Autodesk Inventor part; units mm, degrees
ref_plane "YZ Plane" through (0, 0, 0) normal (1, 0, 0) x (0, 1, 0)
ref_plane "XZ Plane" through (0, 0, 0) normal (0, 1, 0) x (-1, 0, 0)
ref_plane "XY Plane" through (0, 0, 0) normal (0, 0, 1) x (1, 0, 0)
sketch "Szkic1" plane through (0, 0, 0) normal (0, 1, 0) x (-1, 0, 0)
  circle A0 centre (0, 0) radius 10
  dimension "d0" = 20
extrude "Wyciągnięcie proste1" add sketch "Szkic1" along normal mid plane 30
sketch "Szkic2" plane through (0, 15, 0) normal (0, 1, 0) x (1, 0, 0)
  circle A0 centre (0, 0) radius 10
  circle A1 centre (0, 0) radius 15
  dimension "d3" = 30
extrude "Wyciągnięcie proste2" add sketch "Szkic2" along normal blind 5 contours A0 | A1
mirror "Odbicie lustrzane1" about plane through (0, 0, 0) normal (0, 1, 0) of "Wyciągnięcie proste2"
properties part number "RevolvingConnector2" material "Aluminium 6061"
Verification items for the finished model (mm, model axes). A direction names the side the tool comes from. Coordinates: 2 decimals unless noted, no trailing zeros. Write each loop counter-clockwise with the first axis right and the second up, starting at its lowest first coordinate (ties: lowest second). Pieces come first, ordered by that corner, then holes. Notation, with made-up numbers: (39.5, 55) - (55.5, 55) arc R18 cw to (55.5, 85) - close; hole circle Ø6 at (0.5, 68.5). An arc over 180 degrees is marked (long way). Answer as a JSON object with one key per item and string values.
(1) Tool access check on faces 1 (the flat face through (3, 15, 10)), 2 (the cylindrical face through (-14.985, -17.465, -0.66)). Record the directions out of +Z, -Z, +X, -X, +Y, -Y that give a thin tool (end or side, any length) a straight path to the whole face; none if there is none.
Report:
{"face 1": "none", "face 2": "+Y, -Y"}
(2) Cross-section at C-C on z = 0. Record the cut outline in (x, y).
Report:
{"outline": "(-15, -20) - (15, -20) - (15, -15) - (10, -15) - (10, 15) - (15, 15) - (15, 20) - (-15, 20) - (-15, 15) - (-10, 15) - (-10, -15) - (-15, -15) - close"}
(3) Cross-section at D-D on y = -12.5. Record the cut outline in (x, z).
Report:
{"outline": "circle Ø20 at (0, 0)"}
(4) Mould release check, pull along Y, two halves, no side actions. Record for faces 3 (the flat face through (0, 20, 0)), 4 (the flat face through (-3, -15, 10)), 5 (the cylindrical face through (-14.985, 17.465, 0.66)): pulls with the +Y half, pulls with the -Y half, needs draft (parallel to the pull), parting line crosses it, or undercut.
Report:
{"face 3": "pulls with the +Y half", "face 4": "undercut", "face 5": "needs draft"}
(5) Thickness scan on line 1 along Y through (x, z) = (-12, 3.75); line 2 along X through (y, z) = (13, -7.5); line 3 along X through (y, z) = (0, -8). Record the ranges inside material, lowest first.
Report:
{"line 1": "-20 to -15, 15 to 20", "line 2": "-6.61 to 6.61", "line 3": "-6 to 6"}
(6) Gauge pin test, flat ends, axial feed: pin 1 Ø8 at (y, z) = (-8.5, 8) entering from +X; pin 2 Ø2 at (y, z) = (13.5, -10) entering from -X; pin 3 Ø6 at (y, z) = (-7, -8) entering from -X. Record the tip position at first contact, or that the pin passes through.
Report:
{"pin 1": "x = 9.17", "pin 2": "x = -4.36", "pin 3": "x = -8.66"}
(7) Cross-section at B-B on z = -10.75. Record the cut outline in (x, y).
Report:
{"outline": "(-10.46, -20) - (10.46, -20) - (10.46, -15) - (-10.46, -15) - close; (-10.46, 15) - (10.46, 15) - (10.46, 20) - (-10.46, 20) - close"}
(8) Cross-section at A-A on x = 0. Record the cut outline in (y, z).
Report:
{"outline": "(-20, -15) - (-15, -15) - (-15, -10) - (15, -10) - (15, -15) - (20, -15) - (20, 15) - (15, 15) - (15, 10) - (-15, 10) - (-15, 15) - (-20, 15) - close"}
